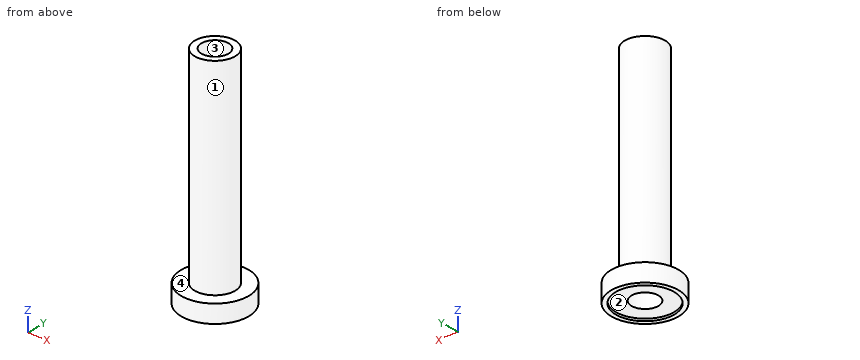
Solid Edge part; units mm, degrees
sketch "Sketch1" plane through (0, 0, 0) normal (0, 0, 1) x (1, 0, 0)
  circle A0 centre (0, 0) radius 7.5
  circle A1 centre (0, 0) radius 3
extrude "Protrusion1" add sketch "Sketch1" along normal blind 50
sketch "Sketch2" plane through (0, 0, 50) normal (0, 0, 1) x (0, -1, 0)
  circle A0 centre (0, 0) radius 4.5
  circle A1 centre (0, 0) radius 7.5
extrude "ExtrudedCutout_1" cut sketch "Sketch2" against normal blind 46
sketch "Sketch3" plane through (0, 0, 0) normal (0, 0, -1) x (0, -1, 0)
  circle A0 centre (0, 0) radius 6.5
extrude "ExtrudedCutout_2" cut sketch "Sketch3" against normal blind 0.5
The model under review builds one solid part; all positions refer to its coordinate system, in mm. Face numbers are marked on the shaded views. Round coordinates to 2 decimals unless told otherwise and drop trailing zeros. Write each loop counter-clockwise with the first axis right and the second up, starting at its lowest first coordinate (ties: lowest second). Pieces come first, ordered by that corner, then holes. Notation, with made-up numbers: (69, 35.25) -> (90, 35.25) arc R10 cw to (90, 46.25) -> close; hole circle Ø7 at (25, 46.5). An arc over 180 degrees is marked (long way). Use CSV: the item, a comma, the result in double quotes.
Q1. For pin 1 Ø3 at (x, y) = (5, -5) entering from +Z; pin 2 Ø3 at (x, z) = (-0.5, 33.5) entering from -Y; pin 3 Ø1.5 at (x, z) = (-0.5, 7.5) entering from +Y, all flat-tipped, find the tip position at first contact; note any pin that passes through.
Checks:
pin 1,"z = 4"
pin 2,"y = -4.5"
pin 3,"y = 4.5"
Q2. Consider section D-D (x = -5.5). Give the boundary of the cut face in (y, z).
Checks:
outline,"(-5.1, 0) -> (-3.46, 0) -> (-3.46, 0.5) -> (3.46, 0.5) -> (3.46, 0) -> (5.1, 0) -> (5.1, 4) -> (-5.1, 4) -> close"
Q3. To check wall thickness, follow probe 1 along X at (y, z) = (0, 0.25); probe 2 along X at (y, z) = (0.25, 30). State the ranges of each line that lie inside material, in increasing order. Write a range as [from, to].
Checks:
probe 1,"[-7.5, -6.5], [6.5, 7.5]"
probe 2,"[-4.49, -2.99], [2.99, 4.49]"
Q4. Consider section A-A (x = 0). Give the boundary of the cut face in (y, z), then the cut area to 4 significant figures.
Checks:
outline,"(-7.5, 0) -> (-6.5, 0) -> (-6.5, 0.5) -> (-3, 0.5) -> (-3, 50) -> (-4.5, 50) -> (-4.5, 4) -> (-7.5, 4) -> close; (3, 0.5) -> (6.5, 0.5) -> (6.5, 0) -> (7.5, 0) -> (7.5, 4) -> (4.5, 4) -> (4.5, 50) -> (3, 50) -> close"
area,"170.5 mm²"
Q5. Mouldability with a two-part tool opening along Y and no side actions: class the marked faces 1, 2, 3 and 4 as released by +Y, released by -Y, zero draft, split by the parting line, or undercut.
Checks:
face 1,"split by the parting line"
face 2,"undercut"
face 3,"undercut"
face 4,"zero draft"
Q6. Consider section C-C (y = 5.75). Give the boundary of the cut face in (x, z).
Checks:
outline,"(-4.82, 0) -> (-3.03, 0) -> (-3.03, 0.5) -> (3.03, 0.5) -> (3.03, 0) -> (4.82, 0) -> (4.82, 4) -> (-4.82, 4) -> close"
